```python
from build123d import *

# Parameters (mm, degrees)
F0_R     = 20
F1_DEPTH = 100
F2_R     = 2.375
F3_DEPTH = 20
F4_R     = 2.375
F5_DEPTH = 40


with BuildPart() as f1:
    # F0 (on Right) → F1 (new body)
    with BuildSketch(Plane.YZ):
        Circle(F0_R)
    extrude(amount=F1_DEPTH)

    # F2 (on face) → F3 (join)
    with BuildSketch(Plane.YZ.offset(100)):
        Circle(F2_R)
    extrude(amount=F3_DEPTH)

    # F4 (on face) → F5 (join)
    with BuildSketch(Plane.YZ):
        Circle(F4_R)
    extrude(amount=-F5_DEPTH)


solid = f1.part
```
The model under review builds one solid part; all positions refer to its coordinate system, in mm. A direction names the side the tool comes from. Coordinates: 2 decimals unless noted, no trailing zeros. Write each loop counter-clockwise with the first axis right and the second up, starting at its lowest first coordinate (ties: lowest second). Pieces come first, ordered by that corner, then holes.
1) We need section D-D on x = 55.5. State the section outline as (y, z) points.
2) Machinability: for faces 1 (the face through (109.86, 1.096, -2.107)), 2 (the face through (120, 0, 0)), 3 (the face through (-19.72, 1.096, -2.107)), which of the approach directions +Z, -Z, +X, -X, +Y, -Y give a long, thin tool a straight path to every point of the face, cutting with its end or side? Answer none if there is none.
3) We need section A-A on z = 0. State the section outline as (x, y) points (3 decimals), then the cut area to 4 significant figures.
4) Clearance check with flat-ended pins moving along their axes: pin 1 Ø12 at (y, z) = (9, -2.5) entering from +X; pin 2 Ø4 at (x, z) = (30.5, -3) entering from +Y (3 decimals); pin 3 Ø2 at (x, y) = (95, 15.5) entering from +Z (3 decimals). State where each tip first meets the part, or that it passes through.
5) To check wall thickness, follow probe 1 along X at (y, z) = (5.5, 13.5); probe 2 along Y at (x, z) = (82.5, 1); probe 3 along Z at (x, y) = (64, -17). State the ranges of each line that lie inside material, in increasing order.
6) We need section C-C on x = -28.5. State the section outline as (y, z) points (3 decimals), then the cut area to 3 significant figures.
Answer list:
1. outline: circle Ø40 at (0, 0)
2. face 1: +X
2. face 2: +Z, -Z, +X, +Y, -Y
2. face 3: -X
3. outline: (-40, -2.375) - (0, -2.375) - (0, -20) - (100, -20) - (100, -2.375) - (120, -2.375) - (120, 2.375) - (100, 2.375) - (100, 20) - (0, 20) - (0, 2.375) - (-40, 2.375) - close
3. area: 4,285 mm2
4. pin 1: stops at x = 100
4. pin 2: stops at y = 19.975
4. pin 3: stops at z = 13.775
5. probe 1: x = 0 to 100
5. probe 2: y = -19.97 to 19.97
5. probe 3: z = -10.54 to 10.54
6. outline: circle Ø4.75 at (0, 0)
6. area: 17.7 mm2
